Check sheet for the modelled part. Datum: model origin and axes. Units: mm. Give positions to 0.01 mm unless a question says otherwise; leave off trailing zeros. Loops run counter-clockwise (first coordinate to the right, second up) from the corner with the lowest first, then second, coordinate; pieces in that order, holes last. Notation, with made-up numbers: (-5.5, 80.25) - (42.5, 80.25) arc R11 cw to (42.5, 92.25) - close; hole circle Ø10 at (-34.75, 11). An arc over 180 degrees is marked (long way). Use CSV: the item, a comma, the result in double quotes.
from build123d import *

# Parameters (mm, degrees)
SKETCH1_R           = 150
BOSS_EXTRUDE1_DEPTH = 6.35
SKETCH2_R           = 1.5875
SKETCH2_W           = 80.264
SKETCH2_H           = 12.954
CUT_EXTRUDE1_DEPTH  = 213.227054119
SKETCH3_R           = 1.5875
CUT_EXTRUDE2_DEPTH  = 213.227054119
SKETCH4_R           = 1.5875
SKETCH4_W           = 46.99
SKETCH4_H           = 138.43
CUT_EXTRUDE3_DEPTH  = 213.227054119


with BuildPart() as part:
    # Sketch1 → Boss-Extrude1 (new body)
    with BuildSketch(Plane(origin=(0, 0, 0), x_dir=(1, 0, 0), z_dir=(0, 1, 0))):
        with Locations(Location((0, 0, 0), (0, 0, 270))):
            Circle(SKETCH1_R)
    extrude(amount=-BOSS_EXTRUDE1_DEPTH)

    # Sketch2 → Cut-Extrude1 (cut, through all)
    with BuildSketch(Plane(origin=(0, 0, 0), x_dir=(1, 0, 0), z_dir=(0, 1, 0))):
        with Locations(Location((36.144045702, -67.691, 0), (0, 0, 270))):
            Circle(SKETCH2_R)
        with Locations(Location((36.144045702, -61.341, 0), (0, 0, 270))):
            Circle(SKETCH2_R)
        with Locations(Location((36.144045702, -54.991, 0), (0, 0, 270))):
            Circle(SKETCH2_R)
        with Locations(Location((36.144045702, -48.641, 0), (0, 0, 270))):
            Circle(SKETCH2_R)
        with Locations(Location((36.144045702, -42.291, 0), (0, 0, 270))):
            Circle(SKETCH2_R)
        with Locations(Location((36.144045702, -35.941, 0), (0, 0, 270))):
            Circle(SKETCH2_R)
        with Locations(Location((36.144045702, -29.591, 0), (0, 0, 270))):
            Circle(SKETCH2_R)
        with Locations(Location((67.894045702, -67.691, 0), (0, 0, 270))):
            Circle(SKETCH2_R)
        with Locations(Location((67.894045702, -61.341, 0), (0, 0, 270))):
            Circle(SKETCH2_R)
        with Locations(Location((67.894045702, -54.991, 0), (0, 0, 270))):
            Circle(SKETCH2_R)
        with Locations(Location((67.894045702, -48.641, 0), (0, 0, 270))):
            Circle(SKETCH2_R)
        with Locations(Location((67.894045702, -42.291, 0), (0, 0, 270))):
            Circle(SKETCH2_R)
        with Locations(Location((67.894045702, -35.941, 0), (0, 0, 270))):
            Circle(SKETCH2_R)
        with Locations(Location((67.894045702, -29.591, 0), (0, 0, 270))):
            Circle(SKETCH2_R)
        with Locations(Location((36.144045702, 67.691, 0), (0, 0, 270))):
            Circle(SKETCH2_R)
        with Locations(Location((36.144045702, 61.341, 0), (0, 0, 270))):
            Circle(SKETCH2_R)
        with Locations(Location((36.144045702, 54.991, 0), (0, 0, 270))):
            Circle(SKETCH2_R)
        with Locations(Location((36.144045702, 48.641, 0), (0, 0, 270))):
            Circle(SKETCH2_R)
        with Locations(Location((36.144045702, 42.291, 0), (0, 0, 270))):
            Circle(SKETCH2_R)
        with Locations(Location((36.144045702, 35.941, 0), (0, 0, 270))):
            Circle(SKETCH2_R)
        with Locations(Location((36.144045702, 29.591, 0), (0, 0, 270))):
            Circle(SKETCH2_R)
        with Locations(Location((67.894045702, 67.691, 0), (0, 0, 270))):
            Circle(SKETCH2_R)
        with Locations(Location((67.894045702, 61.341, 0), (0, 0, 270))):
            Circle(SKETCH2_R)
        with Locations(Location((67.894045702, 54.991, 0), (0, 0, 270))):
            Circle(SKETCH2_R)
        with Locations(Location((67.894045702, 48.641, 0), (0, 0, 270))):
            Circle(SKETCH2_R)
        with Locations(Location((67.894045702, 42.291, 0), (0, 0, 270))):
            Circle(SKETCH2_R)
        with Locations(Location((67.894045702, 35.941, 0), (0, 0, 270))):
            Circle(SKETCH2_R)
        with Locations(Location((67.894045702, 29.591, 0), (0, 0, 270))):
            Circle(SKETCH2_R)
        with Locations((52.019045702, -96.4438)):
            Rectangle(SKETCH2_W, SKETCH2_H)
        with Locations((52.019045702, 96.4438)):
            Rectangle(SKETCH2_W, SKETCH2_H)
    extrude(amount=-CUT_EXTRUDE1_DEPTH, mode=Mode.SUBTRACT)

    # Sketch3 → Cut-Extrude2 (cut, through all)
    with BuildSketch(Plane(origin=(0, 0, 0), x_dir=(1, 0, 0), z_dir=(0, 1, 0))):
        with Locations(Location((-43.611954298, 77.2668, 0), (0, 0, 270))):
            Circle(SKETCH3_R)
        with Locations(Location((22.428045702, 77.2668, 0), (0, 0, 270))):
            Circle(SKETCH3_R)
        with Locations(Location((22.428045702, -34.4932, 0), (0, 0, 270))):
            Circle(SKETCH3_R)
        with Locations(Location((-43.611954298, -34.4932, 0), (0, 0, 270))):
            Circle(SKETCH3_R)
    extrude(amount=-CUT_EXTRUDE2_DEPTH, mode=Mode.SUBTRACT)

    # Sketch4 → Cut-Extrude3 (cut, through all)
    with BuildSketch(Plane(origin=(0, 0, 0), x_dir=(1, 0, 0), z_dir=(0, 1, 0))):
        with Locations(Location((65.354045702, 0, 0), (0, 0, 270))):
            Circle(SKETCH4_R)
        with Locations(Location((138.252045702, 0, 0), (0, 0, 270))):
            Circle(SKETCH4_R)
        with Locations((101.549045702, 0)):
            Rectangle(SKETCH4_W, SKETCH4_H)
    extrude(amount=-CUT_EXTRUDE3_DEPTH, mode=Mode.SUBTRACT)


solid = part.part
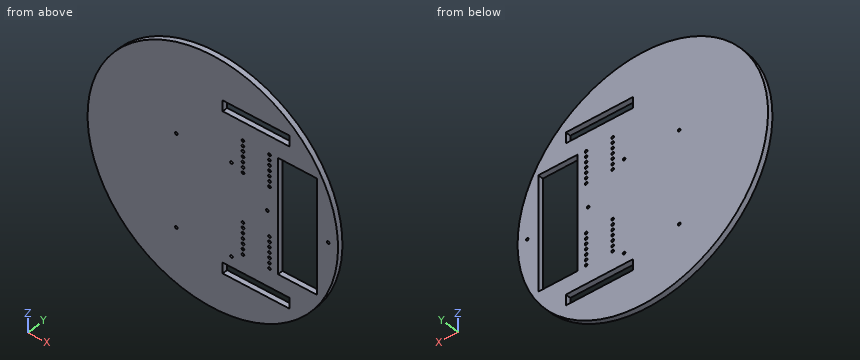
1. Sectioned sample at C-C, the plane x = -81. Record the boundary of the cut face in (y, z).
Completed:
outline,"(-6.35, -126.25) - (0, -126.25) - (0, 126.25) - (-6.35, 126.25) - close"
2. Scan lines: line 1 along Z through (x, y) = (82, -5) (3 decimals); line 2 along X through (y, z) = (-1.75, 0); line 3 along Z through (x, y) = (63, -1). Record each from-to range of solid material in increasing order.
Completed:
line 1,"z = -125.603 to -102.921, -89.967 to -69.215, 69.215 to 89.967, 102.921 to 125.603"
line 2,"x = -150 to 63.77, 66.94 to 78.05, 125.04 to 136.66, 139.84 to 150"
line 3,"z = -136.13 to -102.92, -89.97 to 89.97, 102.92 to 136.13"
3. Sectioned sample at B-B, the plane z = 7.5. Record the boundary of the cut face in (x, y), and give its area (3 significant figures).
Completed:
outline,"(-149.81, -6.35) - (78.05, -6.35) - (78.05, 0) - (-149.81, 0) - close; (125.04, -6.35) - (149.81, -6.35) - (149.81, 0) - (125.04, 0) - close"
area,"1,600 mm²"
4. Go/stop test with flat-tipped pins: pin 1 Ø3 at (y, z) = (-2, 94.5) entering from -X; pin 2 Ø1.9 at (y, z) = (-4.5, -98) entering from +X; pin 3 Ø3 at (y, z) = (-1, 4) entering from +X. Record where each tip stops, or that it passes through.
Completed:
pin 1,"stops at x = -117.69"
pin 2,"stops at x = 114.37"
pin 3,"stops at x = 149.98"
5. Sectioned sample at A-A, the plane x = 16. Record the boundary of the cut face in (y, z).
Completed:
outline,"(-6.35, -149.14) - (0, -149.14) - (0, -102.92) - (-6.35, -102.92) - close; (-6.35, -89.97) - (0, -89.97) - (0, 89.97) - (-6.35, 89.97) - close; (-6.35, 102.92) - (0, 102.92) - (0, 149.14) - (-6.35, 149.14) - close"
6. Sectioned sample at D-D, the plane y = -3.25. State how many separate pieces and enclosed holes the cut face has, and give its area (3 significant figures).
Completed:
separate pieces,"1"
enclosed holes,"37"
area,"61,800 mm²"
